from build123d import *

# Parameters (mm, degrees)
F0_W     = 50.8
F0_H     = 50.8
F0_W_2   = 6.462844
F0_H_2   = 5.558045
F1_DEPTH = 25.4
F2_R     = 9.444234
F3_DEPTH = 25.4
F4_DEPTH = 50.801


with BuildPart() as f1:
    # F0 (on Front) → F1 (new body)
    with BuildSketch(Plane.XZ):
        with Locations((-19.839903, -2.06811)):
            Rectangle(F0_W, F0_H)
        with Locations((-18.225218, 2.779022)):
            Rectangle(F0_W_2, F0_H_2, mode=Mode.SUBTRACT)
    extrude(amount=F1_DEPTH)

    # F2 (on face) → F3 (join)
    with BuildSketch(Plane.XZ.offset(25.4)):
        with Locations((-17.536797, 2.779023)):
            Circle(F2_R)
    extrude(amount=F3_DEPTH)

    # F0 (on Front) → F4 (cut, through all)
    with BuildSketch(Plane.XZ):
        with Locations((-18.225218, 2.779022)):
            Rectangle(F0_W_2, F0_H_2)
    extrude(amount=F4_DEPTH, mode=Mode.SUBTRACT)


solid = f1.part
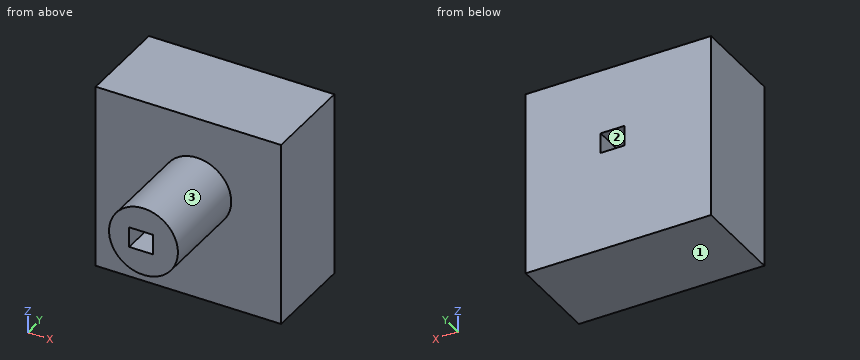
Geometry: final body of the model. Coordinates: model frame, mm. Face numbers are marked on the shaded views. Coordinates: 2 decimals unless noted, no trailing zeros. Order: outer loops, then holes, each group sorted by start corner. A loop starts at its lowest first (then second) coordinate and runs counter-clockwise, first axis right, second up. Notation, with made-up numbers: (27, -10) - (74, -10) arc R27 ccw to (74, 20) - close; hole circle Ø3 at (28.25, -2). An arc over 180 degrees is marked (long way). Use one line per item in the form item = value.
1) Mould query, pull axis Z, two halves, no side actions, for the marked faces 1, 2 and 3. Classes: +Z half, -Z half, draft (parallel to the pull), parting line (faces both ways), or undercut.
Solutions:
face_1 = -Z half
face_2 = undercut
face_3 = parting line
2) Pin query (flat end, axial travel): pin 1 (3 mm diameter, centred on x = -16.5, y = -26, fed in from -Z); pin 2 (5 mm diameter, centred on y = -28.5, z = -1, fed in from +X); pin 3 (4.5 mm diameter, centred on y = -28.5, z = 4, fed in from -X); pin 4 (2 mm diameter, centred on x = -37, z = 9, fed in from -Y). Return the tip coordinate at first contact, or that it passes through.
Solutions:
pin_1 = -27.47
pin_2 = -8.18
pin_3 = -26.98
pin_4 = -25.4
3) Ray query, L1, parallel to Z at x = -17.5, y = -41; L2, parallel to Z at x = -18, y = -7.5; L3, parallel to X at y = -44, z = 5. Return the intervals inside material, ascending.
Solutions:
L1 = -6.67 to 0, 5.56 to 12.22
L2 = -27.47 to 0, 5.56 to 23.33
L3 = -26.72 to -21.46, -14.99 to -8.36
4) Section C-C (y = -40). Return loops of the section in (x, z).
Solutions:
outline = circle Ø18.89 at (-17.54, 2.78); hole (-21.46, 0) - (-14.99, 0) - (-14.99, 5.56) - (-21.46, 5.56) - close
5) Section B-B (x = -20). Return loops of the section in (y, z), then the cut area to 3 significant figures.
Solutions:
outline = (-50.8, -6.34) - (-25.4, -6.34) - (-25.4, -27.47) - (0, -27.47) - (0, 0) - (-50.8, 0) - close; (-50.8, 5.56) - (0, 5.56) - (0, 23.33) - (-25.4, 23.33) - (-25.4, 11.9) - (-50.8, 11.9) - close
area = 1,470 mm^2
6) Section A-A (z = -4.5). Return loops of the section in (x, y), then the cut area to 3 significant figures.
Solutions:
outline = (-45.24, -25.4) - (-23.55, -25.4) - (-23.55, -50.8) - (-11.52, -50.8) - (-11.52, -25.4) - (5.56, -25.4) - (5.56, 0) - (-45.24, 0) - close
area = 1,600 mm^2
7) Section D-D (x = -6). Return loops of the section in (y, z).
Solutions:
outline = (-25.4, -27.47) - (0, -27.47) - (0, 23.33) - (-25.4, 23.33) - close
